from build123d import *

# Parameters (mm, degrees)
F0_R     = 60
F1_DEPTH = 7
F2_SIZE  = 1
F4_D     = 14.5


with BuildPart() as f1:
    # F0 (on Top) → F1 (new body)
    with BuildSketch(Plane.XY):
        Circle(F0_R)
    extrude(amount=F1_DEPTH)

    # F2
    f2_edges = [f1.edges().sort_by_distance(p)[0] for p in [
        (-60, 0, 7),
        (-60, 0, 0),
    ]]
    chamfer(f2_edges, length=F2_SIZE)

    # F4 (through all)
    with Locations(Plane.XY.offset(7)):
        with Locations((0, 27.5), (23.8156986041, -13.75), (-23.8156986041, -13.75)):
            Hole(F4_D / 2)


solid = f1.part
The model under review builds one solid part; all positions refer to its coordinate system, in mm. Round coordinates to 2 decimals unless told otherwise and drop trailing zeros. Write each loop counter-clockwise with the first axis right and the second up, starting at its lowest first coordinate (ties: lowest second). Pieces come first, ordered by that corner, then holes. Notation, with made-up numbers: M 11.25,6.5 L 44.25,6.5 A32 ccw 44.25,32.5 Z; hole C 77,9.5 d10. An arc over 180 degrees is marked long. Use a Markdown table: item, result. Add a question column.
Q1. Insertion check: pin 1 (3 mm diameter, centred on x = 6.5, z = 5.5, fed in from -Y); pin 2 (4 mm diameter, centred on y = -8.5, z = 2.5, fed in from -X); pin 3 (2 mm diameter, centred on x = 43, z = 4.5, fed in from +Y). Each pin has a flat end and moves straight along its axis. Give the tip position at first contact, or say it passes through.
Q2. The part is to be moulded in two halves that separate along Y. For faces 1 (the face through (-1, 1, 7)), 2 (the face through (-59.94, 2.64, 3.46)), 3 (the face through (1.57, 20.42, 3.45)), say which applies: pulls with the +Y half, pulls with the -Y half, needs draft (parallel to the pull), parting line crosses it, or undercut.
Q3. We need section A-A, the plane x = 0. State the section outline as (y, z) points, plus the area to 4 significant figures.
Q4. We need section C-C, the plane y = -13.75. Count the separate pieces of the cut face and the enclosed holes in it, plus the area to 3 significant figures.
Q5. We need section B-B, the plane z = 3.5. State the section outline as (x, y) points, plus the area to 3 significant figures.
Q6. To check wall thickness, follow line 1 (Y direction, x = 0, z = 4.5); line 2 (X direction, y = -9, z = 3.75); line 3 (Y direction, x = 1, z = 6.25). State the ranges of each line that lie inside material, in increasing order.
Findings below:
| question | item | result |
|---|---|---|
| 1 | pin 1 | stops at y = -59.79 |
| 1 | pin 2 | stops at x = -59.65 |
| 1 | pin 3 | stops at y = 42.85 |
| 2 | face 1 | needs draft |
| 2 | face 2 | parting line crosses it |
| 2 | face 3 | undercut |
| 3 | outline | M -60,1 L -59,0 L 20.25,0 L 20.25,7 L -59,7 L -60,6 Z; M 34.75,0 L 59,0 L 60,1 L 60,6 L 59,7 L 34.75,7 Z |
| 3 | area | 736.5 mm² |
| 4 | separate pieces | 3 |
| 4 | enclosed holes | 0 |
| 4 | area | 613 mm² |
| 5 | outline | C 0,0 d120; hole C -23.82,-13.75 d14.5; hole C 0,27.5 d14.5; hole C 23.82,-13.75 d14.5 |
| 5 | area | 10,800 mm² |
| 6 | line 1 | y = -60 to 20.25, 34.75 to 60 |
| 6 | line 2 | x = -59.32 to -29.29, -18.34 to 18.34, 29.29 to 59.32 |
| 6 | line 3 | y = -59.74 to 20.32, 34.68 to 59.74 |
